Design review of the part built by this model. Coordinates are the model's own, in mm. Coordinates: 2 decimals unless noted, no trailing zeros. Write each loop counter-clockwise with the first axis right and the second up, starting at its lowest first coordinate (ties: lowest second). Pieces come first, ordered by that corner, then holes. Notation, with made-up numbers: (-38, 28.25) - (-16, 28.25) arc R17 ccw to (-16, 59.25) - close; hole circle Ø8 at (25, -28.75). An arc over 180 degrees is marked (long way). Answer as a JSON object with one key per item and string values.
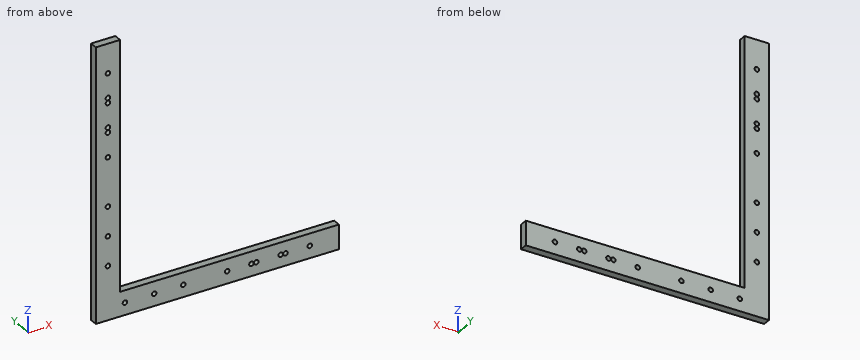
```python
from build123d import *

# Parameters (mm, degrees)
F0_R     = 2.35
F1_DEPTH = 8


with BuildPart() as f1:
    # F0 (on Front) → F1 (new body)
    with BuildSketch(Plane.XZ):
        Polygon((-125, 135), (-125, -145), (125, -145), (125, -120), (-100, -120), (-100, 135), align=None)
        with Locations((-95, -132.5)):
            Circle(F0_R, mode=Mode.SUBTRACT)
        with Locations((-65, -132.5)):
            Circle(F0_R, mode=Mode.SUBTRACT)
        with Locations((-112.5, -90)):
            Circle(F0_R, mode=Mode.SUBTRACT)
        with Locations((-35, -132.5)):
            Circle(F0_R, mode=Mode.SUBTRACT)
        with Locations((-112.5, -60)):
            Circle(F0_R, mode=Mode.SUBTRACT)
        with Locations((-112.5, -30)):
            Circle(F0_R, mode=Mode.SUBTRACT)
        with Locations((10, -132.5)):
            Circle(F0_R, mode=Mode.SUBTRACT)
        with Locations((35, -132.5)):
            Circle(F0_R, mode=Mode.SUBTRACT)
        with Locations((40, -132.5)):
            Circle(F0_R, mode=Mode.SUBTRACT)
        with Locations((65, -132.5)):
            Circle(F0_R, mode=Mode.SUBTRACT)
        with Locations((70, -132.5)):
            Circle(F0_R, mode=Mode.SUBTRACT)
        with Locations((95, -132.5)):
            Circle(F0_R, mode=Mode.SUBTRACT)
        with Locations((-112.5, 20)):
            Circle(F0_R, mode=Mode.SUBTRACT)
        with Locations((-112.5, 45)):
            Circle(F0_R, mode=Mode.SUBTRACT)
        with Locations((-112.5, 50)):
            Circle(F0_R, mode=Mode.SUBTRACT)
        with Locations((-112.5, 75)):
            Circle(F0_R, mode=Mode.SUBTRACT)
        with Locations((-112.5, 80)):
            Circle(F0_R, mode=Mode.SUBTRACT)
        with Locations((-112.5, 105)):
            Circle(F0_R, mode=Mode.SUBTRACT)
    extrude(amount=F1_DEPTH)


solid = f1.part
```
(1) To check wall thickness, follow line 1 (X direction, y = -1, z = -34); line 2 (Z direction, x = 40, y = -6); line 3 (Z direction, x = 1, y = -2.75). State the ranges of each line that lie inside material, in increasing order. Write a range as from..to.
Solved:
{"line 1": "x = -125..-100", "line 2": "z = -145..-134.85, -130.15..-120", "line 3": "z = -145..-120"}
(2) Take a section at C-C, the plane z = 98. Write out the cut boundary in (x, y), and give its area (3 significant figures).
Solved:
{"outline": "(-125, -8) - (-100, -8) - (-100, 0) - (-125, 0) - close", "area": "200 mm^2"}
(3) Take a section at A-A, the plane y = -1.5. Give the number of separate pieces and of enclosed holes in the cut face, and give its area (3 significant figures).
Solved:
{"separate pieces": "1", "enclosed holes": "18", "area": "12,300 mm^2"}
(4) For pin 1 (7.5 mm diameter, centred on x = -112.5, z = 50, fed in from -Y); pin 2 (2 mm diameter, centred on y = -1, z = -63, fed in from +X); pin 3 (2 mm diameter, centred on x = 29.5, y = -1, fed in from +Z), all flat-tipped, find the tip position at first contact; note any pin that passes through.
Solved:
{"pin 1": "stops at y = -8", "pin 2": "stops at x = -100", "pin 3": "stops at z = -120"}
(5) Take a section at B-B, the plane x = -42.5. Write out the cut boundary in (y, z), and give its area (3 significant figures).
Solved:
{"outline": "(-8, -145) - (0, -145) - (0, -120) - (-8, -120) - close", "area": "200 mm^2"}
